from build123d import *

# Parameters (mm, degrees)
SKETCH_1_W          = 63
SKETCH_1_H          = 36
EXTRUDE_1_DEPTH     = 2
SKETCH_2_R          = 3
CUT_EXTRUDE_1_DEPTH = 10
SKETCH_4_W          = 55
SKETCH_4_H          = 36
EXTRUDE_2_DEPTH     = 2
SKETCH_5_R          = 2
CUT_EXTRUDE_2_DEPTH = 37


with BuildPart() as part:
    # 草图1 → 凸台-拉伸1 (new body)
    with BuildSketch(Plane.XY):
        Rectangle(SKETCH_1_W, SKETCH_1_H)
    extrude(amount=EXTRUDE_1_DEPTH)

    # 草图2 → 切除-拉伸1 (cut)
    with BuildSketch(Plane.XY.offset(2)):
        with Locations((-24, 0)):
            Circle(SKETCH_2_R)
        with Locations((24, 0)):
            Circle(SKETCH_2_R)
    extrude(amount=-CUT_EXTRUDE_1_DEPTH, mode=Mode.SUBTRACT)

    # 草图4 → 凸台-拉伸2 (add)
    with BuildSketch(Plane(origin=(0, 18, 0), x_dir=(1, 0, 0), z_dir=(0, 1, 0))):
        with Locations((0, 16)):
            Rectangle(SKETCH_4_W, SKETCH_4_H)
    extrude_2 = extrude(amount=-EXTRUDE_2_DEPTH)

    # 草图5 → 切除-拉伸2 (cut, through all)
    with BuildSketch(Plane(origin=(0, 18, 0), x_dir=(1, 0, 0), z_dir=(0, 1, 0))):
        with Locations((-14.5, 21.5)):
            Circle(SKETCH_5_R)
        with Locations((14.5, 21.5)):
            Circle(SKETCH_5_R)
    cut_extrude_2 = extrude(amount=-CUT_EXTRUDE_2_DEPTH, mode=Mode.SUBTRACT)

    # 镜向1: 凸台-拉伸2, 切除-拉伸2 across plane
    add(extrude_2.mirror(Plane.ZX))
    add(cut_extrude_2.mirror(Plane.ZX), mode=Mode.SUBTRACT)


solid = part.part
Geometry check sheet. Reference: the model listing, model coordinates, mm. A direction names the side the tool comes from. Give positions to 0.01 mm unless a question says otherwise; leave off trailing zeros. Order: outer loops, then holes, each group sorted by start corner. A loop starts at its lowest first (then second) coordinate and runs counter-clockwise, first axis right, second up.
1) Tool access check on faces 4 (the flat face through (-27.5, -17, -17)), 5 (the flat face through (27.5, -17, -17)), 6 (the flat face through (0, -16, -17)), 7 (the cylindrical face through (-14.76, -17.014, -23.483)), 8 (the flat face through (31.5, 0, 1)). Record the directions out of +Z, -Z, +X, -X, +Y, -Y that give a thin tool (end or side, any length) a straight path to the whole face; none if there is none.
Results are:
face 4: -Z, -X, +Y, -Y
face 5: -Z, +X, +Y, -Y
face 6: -Z, +X, -X
face 7: +Y, -Y
face 8: +Z, -Z, +X, +Y, -Y
2) Cross-section at D-D (z = -4). Record the boundary of the cut face in (x, y), then the cut area to 3 significant figures.
Results are:
outline: (-27.5, -18) - (27.5, -18) - (27.5, -16) - (-27.5, -16) - close; (-27.5, 16) - (27.5, 16) - (27.5, 18) - (-27.5, 18) - close
area: 220 mm2
3) Cross-section at B-B (y = 0). Record the boundary of the cut face in (x, z), then the cut area to 3 significant figures.
Results are:
outline: (-31.5, 0) - (-27, 0) - (-27, 2) - (-31.5, 2) - close; (-21, 0) - (21, 0) - (21, 2) - (-21, 2) - close; (27, 0) - (31.5, 0) - (31.5, 2) - (27, 2) - close
area: 102 mm2
4) Draft check along Z on faces 1 (the cylindrical face through (13.026, -17.014, -22.852)), 2 (the flat face through (0, -17, -34)), 3 (the flat face through (0, 16, -17)). Enter one of: released by +Z, released by -Z, zero draft, split by the parting line, or undercut.
Results are:
face 1: undercut
face 2: released by -Z
face 3: zero draft
5) Material ranges on probe 1 along X at (y, z) = (17.25, -21.5); probe 2 along Y at (x, z) = (-10, -30.5); probe 3 along Z at (x, y) = (14.5, -16.8), recorded low to high.
Results are:
probe 1: x = -27.5 to -16.5, -12.5 to 12.5, 16.5 to 27.5
probe 2: y = -18 to -16, 16 to 18
probe 3: z = -34 to -23.5, -19.5 to 2
6) Gauge pin test, flat ends, axial feed: pin 1 (3.5 mm diameter, centred on x = 24, y = 0, fed in from -Z); pin 2 (6.5 mm diameter, centred on x = 14.5, z = -21.5, fed in from +Y); pin 3 (2 mm diameter, centred on y = -17, z = -16, fed in from -X); pin 4 (5 mm diameter, centred on x = 22, y = 11, fed in from -Z). Record the tip position at first contact, or that the pin passes through.
Results are:
pin 1: passes through
pin 2: stops at y = 18
pin 3: stops at x = -27.5
pin 4: stops at z = 0
7) Cross-section at C-C (z = -21.5). Record the boundary of the cut face in (x, y).
Results are:
outline: (-27.5, -18) - (-16.5, -18) - (-16.5, -16) - (-27.5, -16) - close; (-27.5, 16) - (-16.5, 16) - (-16.5, 18) - (-27.5, 18) - close; (-12.5, -18) - (12.5, -18) - (12.5, -16) - (-12.5, -16) - close; (-12.5, 16) - (12.5, 16) - (12.5, 18) - (-12.5, 18) - close; (16.5, -18) - (27.5, -18) - (27.5, -16) - (16.5, -16) - close; (16.5, 16) - (27.5, 16) - (27.5, 18) - (16.5, 18) - close
8) Cross-section at A-A (x = 24). Record the boundary of the cut face in (y, z), then the cut area to 3 significant figures.
Results are:
outline: (-18, -34) - (-16, -34) - (-16, 0) - (-3, 0) - (-3, 2) - (-18, 2) - close; (3, 0) - (16, 0) - (16, -34) - (18, -34) - (18, 2) - (3, 2) - close
area: 196 mm2
